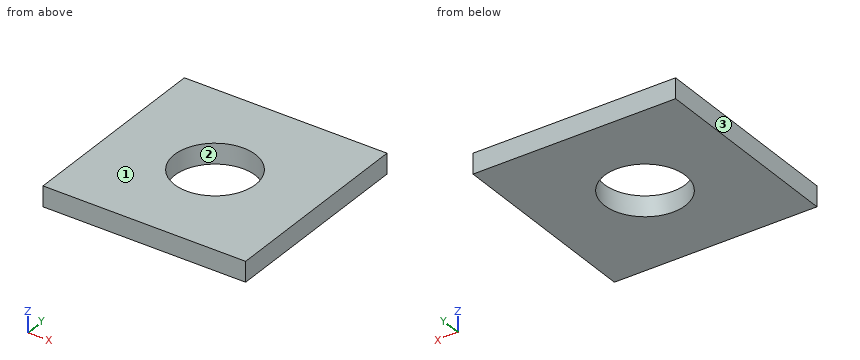
from build123d import *

# Parameters (mm, degrees)
CROQUIS1_W              = 100
CROQUIS1_H              = 100
SALIENTE_EXTRUIR1_DEPTH = 10
CORTAR_EXTRUIR1_REACH   = 73.414
CROQUIS2_R              = 20


with BuildPart() as part:
    # Croquis1 → Saliente-Extruir1 (new body)
    with BuildSketch(Plane.XY):
        Rectangle(CROQUIS1_W, CROQUIS1_H)
    extrude(amount=SALIENTE_EXTRUIR1_DEPTH)

    # Croquis2 → Cortar-Extruir1 (cut, up to next)
    with BuildSketch(Plane.XY.offset(10), mode=Mode.PRIVATE) as cortar_extruir1_sk1:
        Circle(CROQUIS2_R)
    cortar_extruir1_tool1 = extrude(cortar_extruir1_sk1.sketch, amount=-CORTAR_EXTRUIR1_REACH, mode=Mode.PRIVATE) & part.part
    add(cortar_extruir1_tool1.solids().sort_by_distance((0, 0, 10))[0], mode=Mode.SUBTRACT)


solid = part.part
Model file for the job. Use its own axes, mm. Face numbers are marked on the shaded views. Coordinates: 2 decimals unless noted, no trailing zeros. Write each loop counter-clockwise with the first axis right and the second up, starting at its lowest first coordinate (ties: lowest second). Pieces come first, ordered by that corner, then holes. Notation, with made-up numbers: (-34.75, 87) - (-13.75, 87) arc R31 ccw to (-13.75, 113) - close; hole circle Ø5 at (0, 26). An arc over 180 degrees is marked (long way). Write each question's results on one line, items separated by ' | '. Start each with the question number.
1) Cut at C-C (z = 7). Write the cut outline in (x, y), then the cut area to 3 significant figures.
2) Probe line 1 along Y through (x, z) = (0, 6); line 2 along Y through (x, z) = (-3.5, 2.75). List the from-to ranges inside material, lowest first. Write a range as from..to.
3) Mould opens along X. For the marked faces 1, 2 and 3 say: pulls with the +X half, pulls with the -X half, needs draft (parallel to the pull), parting line crosses it, or undercut.
4) Cut at A-A (y = 0). Write the cut outline in (x, z), then the cut area to 3 significant figures.
Returned:
1) outline: (-50, -50) - (50, -50) - (50, 50) - (-50, 50) - close; hole circle Ø40 at (0, 0) | area: 8,740 mm^2
2) line 1: -50..-20, 20..50 | line 2: -50..-19.69, 19.69..50
3) face 1: needs draft | face 2: undercut | face 3: pulls with the -X half
4) outline: (-50, 0) - (-20, 0) - (-20, 10) - (-50, 10) - close; (20, 0) - (50, 0) - (50, 10) - (20, 10) - close | area: 600 mm^2
